```python
from build123d import *

# Parameters (mm, degrees)
F2_R     = 17.016537
F3_DEPTH = 25.4
F1_R     = 30.280081
F4_DEPTH = 11.43
F0_R     = 41.181284
F5_DEPTH = 3.556


with BuildPart() as f3:
    # F2 (on Front) → F3 (new body)
    with BuildSketch(Plane.XZ):
        Circle(F2_R)
    extrude(amount=F3_DEPTH)

    # F1 (on Front) → F4 (join)
    with BuildSketch(Plane.XZ):
        Circle(F1_R)
    extrude(amount=F4_DEPTH)

    # F0 (on Front) → F5 (join)
    with BuildSketch(Plane.XZ):
        Circle(F0_R)
    extrude(amount=F5_DEPTH)


solid = f3.part
```
The model under review builds one solid part; all positions refer to its coordinate system, in mm. Coordinates: 2 decimals unless noted, no trailing zeros. Write each loop counter-clockwise with the first axis right and the second up, starting at its lowest first coordinate (ties: lowest second). Pieces come first, ordered by that corner, then holes. Notation, with made-up numbers: (-31, 49.5) - (5, 49.5) arc R30 ccw to (5, 83.5) - close; hole circle Ø6 at (79, 34). An arc over 180 degrees is marked (long way). Answer in a Markdown table with one row per item. Add a question column.
Q1. Consider section B-B on x = 0. Give the boundary of the cut face in (y, z).
Q2. Consider section C-C on y = -22. Give the boundary of the cut face in (x, z).
Q3. Clearance check with flat-ended pins moving along their axes: pin 1 (8 mm diameter, centred on x = 19.5, y = -18.5, fed in from -Z); pin 2 (3 mm diameter, centred on x = 14, y = -7.5, fed in from -Z); pin 3 (6 mm diameter, centred on y = -3.5, z = -11, fed in from -X). State where each tip first meets the part, or that it passes through.
Q4. Consider section D-D on z = 26. Give the boundary of the cut face in (x, y).
Q5. To check wall thickness, follow line 1 along Y through (x, z) = (6, -25); line 2 along Y through (x, z) = (29, -12); line 3 along Z through (x, y) = (22.5, -7.5). State the ranges of each line that lie inside material, in increasing order. Write a range as from..to.
Q6. Draft analysis for pull direction Y (two halves, no side actions). For faces 1 (the face through (-1, 0, 1)), 2 (the face through (0, -25.4, 0)), 3 (the face through (-8.93, -1.75, -40.2)), state which applies: +Y half, -Y half, draft (parallel to the pull), parting line (faces both ways), or undercut.
Q7. Consider section A-A on z = 0. Give the boundary of the cut face in (x, y), then the cut area to 3 significant figures.
Answers below:
| question | item | result |
|---|---|---|
| 1 | outline | (-25.4, -17.02) - (-11.43, -17.02) - (-11.43, -30.28) - (-3.56, -30.28) - (-3.56, -41.18) - (0, -41.18) - (0, 41.18) - (-3.56, 41.18) - (-3.56, 30.28) - (-11.43, 30.28) - (-11.43, 17.02) - (-25.4, 17.02) - close |
| 2 | outline | circle Ø34.03 at (0, 0) |
| 3 | pin 1 | z = -7.02 |
| 3 | pin 2 | z = -27.58 |
| 3 | pin 3 | x = -40.4 |
| 4 | outline | (-31.94, -3.56) - (-15.52, -3.56) - (-15.52, -11.43) - (15.52, -11.43) - (15.52, -3.56) - (31.94, -3.56) - (31.94, 0) - (-31.94, 0) - close |
| 5 | line 1 | -11.43..0 |
| 5 | line 2 | -3.56..0 |
| 5 | line 3 | -20.26..20.26 |
| 6 | face 1 | +Y half |
| 6 | face 2 | -Y half |
| 6 | face 3 | draft |
| 7 | outline | (-41.18, -3.56) - (-30.28, -3.56) - (-30.28, -11.43) - (-17.02, -11.43) - (-17.02, -25.4) - (17.02, -25.4) - (17.02, -11.43) - (30.28, -11.43) - (30.28, -3.56) - (41.18, -3.56) - (41.18, 0) - (-41.18, 0) - close |
| 7 | area | 1,250 mm² |
